Geometry: final body of the model. Coordinates: model frame, mm. Face numbers are marked on the shaded views. A direction names the side the tool comes from. Round coordinates to 2 decimals unless told otherwise and drop trailing zeros. Loops run counter-clockwise (first coordinate to the right, second up) from the corner with the lowest first, then second, coordinate; pieces in that order, holes last. Notation, with made-up numbers: (33, 40) - (78, 40) arc R31 ccw to (78, 64) - close; hole circle Ø10 at (-25.75, -1). An arc over 180 degrees is marked (long way). Return JSON: item names as keys, results as strings. Group by question number.
1. Material intervals for probe 1 along Y at (x, z) = (-19, -10.25); probe 2 along X at (y, z) = (13, -6); probe 3 along Y at (x, z) = (1.5, 21), sorted ascending.
2. Section A-A on x = -19. Return loops of the section in (y, z).
3. Section D-D on x = 32. Return loops of the section in (y, z).
4. Section C-C on y = 26. Return loops of the section in (x, z), and give its area (3 significant figures).
5. Section B-B on z = -1.5. Return loops of the section in (x, y), and give its area (3 significant figures).
6. Set-up query: the marked faces 1, 2 and 3. Return all of +Z, -Z, +X, -X, +Y, -Y with unobstructed straight access to the full face (end or side cutting, diameter ignored); none if empty.
7. First-contact query: pin 1 Ø2.5 at (x, y) = (-18.5, 21) entering from -Z; pin 2 Ø1.5 at (y, z) = (24.5, 13) entering from -X; pin 3 Ø12 at (x, y) = (-24.5, 18) entering from +Z; pin 4 Ø10 at (x, y) = (-39.5, 19) entering from -Z. Flat tips, straight axial feed; report the tip coordinate or a pass-through.
from build123d import *

# Parameters (mm, degrees)
SKETCH1_W           = 100
SKETCH1_H           = 50
BOSS_EXTRUDE1_DEPTH = 10
CHAMFER1_SIZE       = 10
SKETCH2_W           = 8
SKETCH2_H           = 30
BOSS_EXTRUDE2_DEPTH = 25
SKETCH3_W           = 24.32534271
SKETCH3_H           = 16
CUT_EXTRUDE1_DEPTH  = 10
SKETCH4_R           = 2.5
CUT_EXTRUDE2_DEPTH  = 42


with BuildPart() as part:
    # Sketch1 → Boss-Extrude1 (new body)
    with BuildSketch(Plane(origin=(0, 0, 0), x_dir=(1, 0, 0), z_dir=(0, 1, 0))):
        Rectangle(SKETCH1_W, SKETCH1_H)
    extrude(amount=BOSS_EXTRUDE1_DEPTH)

    # Chamfer1
    chamfer1_edges = [part.edges().sort_by_distance(p)[0] for p in [
        (-50, 5, -25),
        (50, 5, -25),
        (50, 5, 25),
        (-50, 5, 25),
    ]]
    chamfer(chamfer1_edges, length=CHAMFER1_SIZE)

    # Sketch2 → Boss-Extrude2 (add)
    with BuildSketch(Plane(origin=(0, 10, 0), x_dir=(1, 0, 0), z_dir=(0, 1, 0))):
        with Locations((-19, 0)):
            Rectangle(SKETCH2_W, SKETCH2_H)
    extrude(amount=BOSS_EXTRUDE2_DEPTH)

    # Sketch3 → Cut-Extrude1 (cut)
    with BuildSketch(Plane(origin=(0, 35, 0), x_dir=(1, 0, 0), z_dir=(0, 1, 0))):
        with Locations((-18.085363493, 0)):
            Rectangle(SKETCH3_W, SKETCH3_H)
    extrude(amount=-CUT_EXTRUDE1_DEPTH, mode=Mode.SUBTRACT)

    # Sketch4 → Cut-Extrude2 (cut)
    with BuildSketch(Plane.XY.offset(15)):
        with Locations((-19, 30.428638458)):
            Circle(SKETCH4_R)
    extrude(amount=-CUT_EXTRUDE2_DEPTH, mode=Mode.SUBTRACT)


solid = part.part
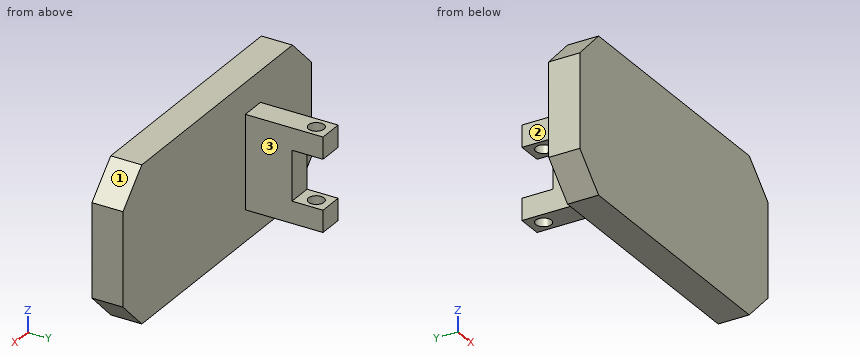
Taken from the geometry:
{
 "1": {"probe 1": "0 to 27.93, 32.93 to 35", "probe 2": "-23 to -15", "probe 3": "0 to 10"},
 "2": {"outline": "(0, -25) - (10, -25) - (10, -15) - (27.93, -15) - (27.93, -8) - (25, -8) - (25, 8) - (27.93, 8) - (27.93, 15) - (10, 15) - (10, 25) - (0, 25) - close; (32.93, -15) - (35, -15) - (35, -8) - (32.93, -8) - close; (32.93, 8) - (35, 8) - (35, 15) - (32.93, 15) - close"},
 "3": {"outline": "(0, -25) - (10, -25) - (10, 25) - (0, 25) - close"},
 "4": {"outline": "(-23, -15) - (-15, -15) - (-15, -8) - (-23, -8) - close; (-23, 8) - (-15, 8) - (-15, 15) - (-23, 15) - close", "area": "112 mm2"},
 "5": {"outline": "(-50, 0) - (50, 0) - (50, 10) - (-15, 10) - (-15, 25) - (-23, 25) - (-23, 10) - (-50, 10) - close", "area": "1,120 mm2"},
 "6": {"face 1": "+Z, +X, +Y, -Y", "face 2": "+Z, -Z, -X, +Y", "face 3": "+Z, -Z, +X, +Y"},
 "7": {"pin 1": "z = -15", "pin 2": "x = -23", "pin 3": "z = 15", "pin 4": "through"}
}
